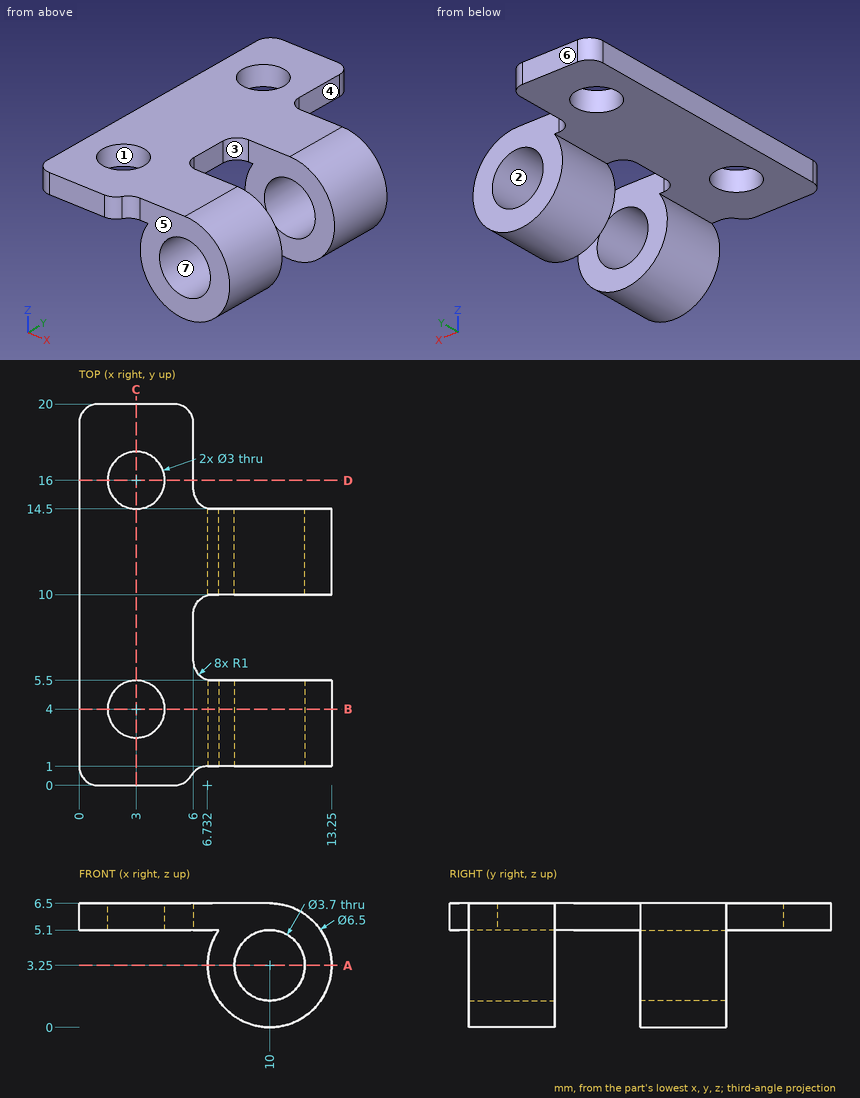
Study the drawing (mm; zero at the part's minimum x, y, z) and answer. A direction names the side the tool comes from. Round coordinates to 2 decimals unless told otherwise and drop trailing zeros. Write each loop counter-clockwise with the first axis right and the second up, starting at its lowest first coordinate (ties: lowest second). Pieces come first, ordered by that corner, then holes. Notation, with made-up numbers: (59.25, 35) - (84.25, 35) arc R19 ccw to (84.25, 56) - close; hole circle Ø8 at (51, 88). An arc over 180 degrees is marked (long way). Use a Markdown table: item, result. Add a question column.
1. The part is cut by section A-A (z = 3.25). Write down the section's boundary in (x, y), and give its area (3 significant figures).
2. The part is cut by section C-C (x = 3). Write down the section's boundary in (y, z).
3. A tool of negligible diameter and unlimited length cuts with its end or side. For the marked faces 1, 2, 3, 4 and 5, from which of +Z, -Z, +X, -X, +Y, -Y can it reach the whole face along a straight path? Write none if from no direction.
4. The part is cut by section B-B (y = 4). Write down the section's boundary in (x, z), and give its area (3 significant figures).
5. The part is cut by section D-D (y = 16). Write down the section's boundary in (x, z), and give its area (3 significant figures).
6. Flat-ended cylindrical pins translate along their axes: P1, Ø1.5, axis at y = 18, z = 5.5, coming from the +X side; P2, Ø2, axis at x = 3, y = 7.5, coming from the -Z side; P3, Ø3, axis at x = 10.5, z = 4, coming from the +Y side. Find the tip coordinate at first contact, or state that the pin passes through.
7. For a pull along Z with two mould halves and no side action, classify the marked faces 6 and 7 as +Z half, -Z half, draft (parallel to the pull), parting line (faces both ways), or undercut.
8. Consider line 1 (Y direction, x = 3, z = 5.7); line 2 (Y direction, x = 8.25, z = 1.75); line 3 (X direction, y = 12.95, z = 3.25). Determine where each line is inside the solid, lowest interval first.
Reported:
| question | item | result |
|---|---|---|
| 1 | outline | (6.75, 1) - (8.15, 1) - (8.15, 5.5) - (6.75, 5.5) - close; (6.75, 10) - (8.15, 10) - (8.15, 14.5) - (6.75, 14.5) - close; (11.85, 1) - (13.25, 1) - (13.25, 5.5) - (11.85, 5.5) - close; (11.85, 10) - (13.25, 10) - (13.25, 14.5) - (11.85, 14.5) - close |
| 1 | area | 25.2 mm^2 |
| 2 | outline | (0, 5.1) - (2.5, 5.1) - (2.5, 6.5) - (0, 6.5) - close; (5.5, 5.1) - (14.5, 5.1) - (14.5, 6.5) - (5.5, 6.5) - close; (17.5, 5.1) - (20, 5.1) - (20, 6.5) - (17.5, 6.5) - close |
| 3 | face 1 | +Z, -Z |
| 3 | face 2 | +Y, -Y |
| 3 | face 3 | +Z, -Z, +X |
| 3 | face 4 | +Z, -Z, +X, +Y |
| 3 | face 5 | +Z, -Z, +X, -Y |
| 4 | outline | (0, 5.1) - (1.5, 5.1) - (1.5, 6.5) - (0, 6.5) - close; (4.5, 5.1) - (7.33, 5.1) arc R3.25 ccw (long way) to (10, 6.5) - (4.5, 6.5) - close; hole circle Ø3.7 at (10, 3.25) |
| 4 | area | 29.6 mm^2 |
| 5 | outline | (0, 5.1) - (1.5, 5.1) - (1.5, 6.5) - (0, 6.5) - close; (4.5, 5.1) - (6, 5.1) - (6, 6.5) - (4.5, 6.5) - close |
| 5 | area | 4.20 mm^2 |
| 6 | P1 | x = 6 |
| 6 | P2 | z = 5.1 |
| 6 | P3 | y = 14.5 |
| 7 | face 6 | draft |
| 7 | face 7 | undercut |
| 8 | line 1 | 0 to 2.5, 5.5 to 14.5, 17.5 to 20 |
| 8 | line 2 | 1 to 5.5, 10 to 14.5 |
| 8 | line 3 | 6.75 to 8.15, 11.85 to 13.25 |
